from build123d import *

# Parameters (mm, degrees)
F0_R     = 39
F0_R_2   = 10.5
F1_DEPTH = 2
F2_R     = 12
F2_R_2   = 10.5
F3_DEPTH = 62
F4_R     = 39
F4_R_2   = 6
F5_DEPTH = 2


with BuildPart() as f1:
    # F0 (on Front) → F1 (new body)
    with BuildSketch(Plane.XZ):
        Circle(F0_R)
        Circle(F0_R_2, mode=Mode.SUBTRACT)
    extrude(amount=F1_DEPTH)

    # F2 (on face) → F3 (join)
    with BuildSketch(Plane.XZ.offset(2)):
        Circle(F2_R)
        Circle(F2_R_2, mode=Mode.SUBTRACT)
    extrude(amount=F3_DEPTH)

    # F4 (on face) → F5 (join)
    with BuildSketch(Plane.XZ.offset(64)):
        Circle(F4_R)
        Circle(F4_R_2, mode=Mode.SUBTRACT)
    extrude(amount=F5_DEPTH)


solid = f1.part
Work out the finished part from the listing and answer in its coordinate system (mm). A direction names the side the tool comes from. Give positions to 0.01 mm unless a question says otherwise; leave off trailing zeros. Loops run counter-clockwise (first coordinate to the right, second up) from the corner with the lowest first, then second, coordinate; pieces in that order, holes last. Notation, with made-up numbers: (39, 77) -> (93, 77) arc R15 cw to (93, 83) -> close; hole circle Ø10 at (-5.75, 49.25). An arc over 180 degrees is marked (long way). Use a Markdown table: item, result. Add a question column.
1. Section B-B on z = 0 is taken. Determine the outline of the cut face in (x, y).
2. Section D-D on x = 26 is taken. Determine the outline of the cut face in (y, z), and give its area (3 significant figures).
3. Determine the mould class of faces 4 (the cylindrical face through (-5.077, -64.986, 38.668)), 5 (the flat face through (5, -64, -5)), 6 (the flat face through (8.1, -64, 9.2)) for opening direction Z: released by +Z, released by -Z, zero draft, split by the parting line, or undercut.
4. Flat-ended cylindrical pins translate along their axes: pin 1 Ø12 at (x, y) = (16, -28) entering from +Z; pin 2 Ø6 at (x, y) = (7.5, -17.5) entering from -Z; pin 3 Ø5 at (x, y) = (-13.5, -59.5) entering from -Z. Find the tip coordinate at first contact, or state that the pin passes through.
5. For faces 1 (the flat face through (8.1, -2, 9.2)), 2 (the flat face through (-1, -66, -8)), 3 (the cylindrical face through (10, -31.6, 3.2)), determine the directions among +Z, -Z, +X, -X, +Y, -Y from which every point of the face is accessible in a straight line to the end or side of a thin tool.
6. Section A-A on x = 0 is taken. Determine the outline of the cut face in (y, z), and give its area (3 significant figures).
7. Section C-C on y = -47.5 is taken. Determine the outline of the cut face in (x, z), and give its area (3 significant figures).
8. Find the intervals of material crossed by probe 1 along Z at (x, y) = (0, -49); probe 2 along Y at (x, z) = (21, -17); probe 3 along Z at (x, y) = (0, -65.25), in increasing order.
Results below:
| question | item | result |
|---|---|---|
| 1 | outline | (-39, -66) -> (-6, -66) -> (-6, -64) -> (-10.5, -64) -> (-10.5, 0) -> (-39, 0) -> (-39, -2) -> (-12, -2) -> (-12, -64) -> (-39, -64) -> close; (6, -66) -> (39, -66) -> (39, -64) -> (12, -64) -> (12, -2) -> (39, -2) -> (39, 0) -> (10.5, 0) -> (10.5, -64) -> (6, -64) -> close |
| 2 | outline | (-66, -29.07) -> (-64, -29.07) -> (-64, 29.07) -> (-66, 29.07) -> close; (-2, -29.07) -> (0, -29.07) -> (0, 29.07) -> (-2, 29.07) -> close |
| 2 | area | 233 mm^2 |
| 3 | face 4 | split by the parting line |
| 3 | face 5 | undercut |
| 3 | face 6 | zero draft |
| 4 | pin 1 | stops at z = 6.63 |
| 4 | pin 2 | stops at z = -11.12 |
| 4 | pin 3 | stops at z = -4.8 |
| 5 | face 1 | none |
| 5 | face 2 | +Z, -Z, +X, -X, -Y |
| 5 | face 3 | +Y |
| 6 | outline | (-66, -39) -> (-64, -39) -> (-64, -12) -> (-2, -12) -> (-2, -39) -> (0, -39) -> (0, -10.5) -> (-64, -10.5) -> (-64, -6) -> (-66, -6) -> close; (-66, 6) -> (-64, 6) -> (-64, 10.5) -> (0, 10.5) -> (0, 39) -> (-2, 39) -> (-2, 12) -> (-64, 12) -> (-64, 39) -> (-66, 39) -> close |
| 6 | area | 432 mm^2 |
| 7 | outline | circle Ø24 at (0, 0); hole circle Ø21 at (0, 0) |
| 7 | area | 106 mm^2 |
| 8 | probe 1 | z = -12 to -10.5, 10.5 to 12 |
| 8 | probe 2 | y = -66 to -64, -2 to 0 |
| 8 | probe 3 | z = -39 to -6, 6 to 39 |
